Check sheet for the modelled part. Datum: model origin and axes. Units: mm. A direction names the side the tool comes from. Coordinates: 2 decimals unless noted, no trailing zeros. Order: outer loops, then holes, each group sorted by start corner. A loop starts at its lowest first (then second) coordinate and runs counter-clockwise, first axis right, second up.
from build123d import *

# Parameters (mm, degrees)
BOSS_EXTRUDE1_DEPTH        = 8
F_12_0_12_DIAMETER_HOLE1_D = 12
SKETCH8_R                  = 5
BOSS_EXTRUDE2_DEPTH        = 45
FILLET1_R                  = 5


with BuildPart() as part:
    # Sketch1 → Boss-Extrude1 (new body)
    with BuildSketch(Plane(origin=(0, 0, 0), x_dir=(1, 0, 0), z_dir=(0, 1, 0))):
        Polygon((-65.68627451, 247.111542704), (18.954741642, 100.509002326), (-150.327290661, 100.509002326), align=None)
    extrude(amount=BOSS_EXTRUDE1_DEPTH)

    # Ø12.0 (12) Diameter Hole1 (through all)
    with Locations(Plane(origin=(0, 8, 0), x_dir=(1, 0, 0), z_dir=(0, 1, 0))):
        with Locations((-65.68627451, 207.111542704), (-115.68627451, 120.509002326), (-15.68627451, 120.509002326)):
            Hole(F_12_0_12_DIAMETER_HOLE1_D / 2)

    # Sketch8 → Boss-Extrude2 (add)
    with BuildSketch(Plane(origin=(0, 0, 0), x_dir=(-1, 0, 0), z_dir=(0, -1, 0))):
        with Locations(Location((65.68627451, 149.376515785, 0), (0, 0, 90))):
            Circle(SKETCH8_R)
    extrude(amount=-BOSS_EXTRUDE2_DEPTH)

    # Fillet1
    fillet1_edges = [part.edges().sort_by_distance(p)[0] for p in [
        (-150.327290661, 4, -100.509002326),
        (18.954741642, 4, -100.509002326),
        (-65.68627451, 4, -247.111542704),
    ]]
    fillet(fillet1_edges, radius=FILLET1_R)


solid = part.part
(1) Thickness scan on probe 1 along Y at (x, z) = (-9, -107.5); probe 2 along X at (y, z) = (7, -108); probe 3 along X at (y, z) = (20.5, -149). Record the ranges inside material, lowest first.
Filled in:
probe 1: y = 0 to 8
probe 2: x = -146 to 14.63
probe 3: x = -70.67 to -60.7
(2) Go/stop test with flat-tipped pins: P1, Ø7, axis at x = -65.69, z = -207.11, coming from the +Y side; P2, Ø19, axis at x = -15.69, z = -120.51, coming from the +Y side. Record where each tip stops, or that it passes through.
Filled in:
P1: passes through
P2: stops at y = 8
(3) Cross-section at B-B (x = -13). Enter the section's corners in (y, z), and give its area (3 significant figures).
Filled in:
outline: (0, -155.86) - (8, -155.86) - (8, -125.87) - (0, -125.87) - close; (0, -115.14) - (8, -115.14) - (8, -100.51) - (0, -100.51) - close
area: 357 mm2
(4) Release check for a two-part mould opening along X. For faces 3 (the cylindrical face through (14.66, 4.06, -103.07)), 4 (the cylindrical face through (-65.61, 4.06, -242.11)), 5 (the cylindrical face through (-64.91, 3.94, -213.06)), 6 (the flat face through (-65, 0, -155)) record: +X half, -X half, draft (parallel to the pull), parting line (faces both ways), or undercut.
Filled in:
face 3: +X half
face 4: parting line
face 5: undercut
face 6: draft
(5) Cross-section at A-A (x = -111.5). Enter the section's corners in (y, z), and give its area (3 significant figures).
Filled in:
outline: (0, -167.76) - (8, -167.76) - (8, -124.81) - (0, -124.81) - close; (0, -116.21) - (8, -116.21) - (8, -100.51) - (0, -100.51) - close
area: 469 mm2
(6) Cross-section at D-D (y = 14.5). Enter the section's corners in (x, z).
Filled in:
outline: circle Ø10 at (-65.69, -149.38)
(7) Cross-section at C-C (z = -182). Enter the section's corners in (x, y), and give its area (3 significant figures).
Filled in:
outline: (-103.28, 0) - (-28.09, 0) - (-28.09, 8) - (-103.28, 8) - close
area: 601 mm2
(8) Tool access check on faces 1 (the cylindrical face through (-60.73, 26.24, -148.73)), 2 (the flat face through (-66, 45, -149)). Record the directions out of +Z, -Z, +X, -X, +Y, -Y that give a thin tool (end or side, any length) a straight path to the whole face; none if there is none.
Filled in:
face 1: +Y
face 2: +Z, -Z, +X, -X, +Y
